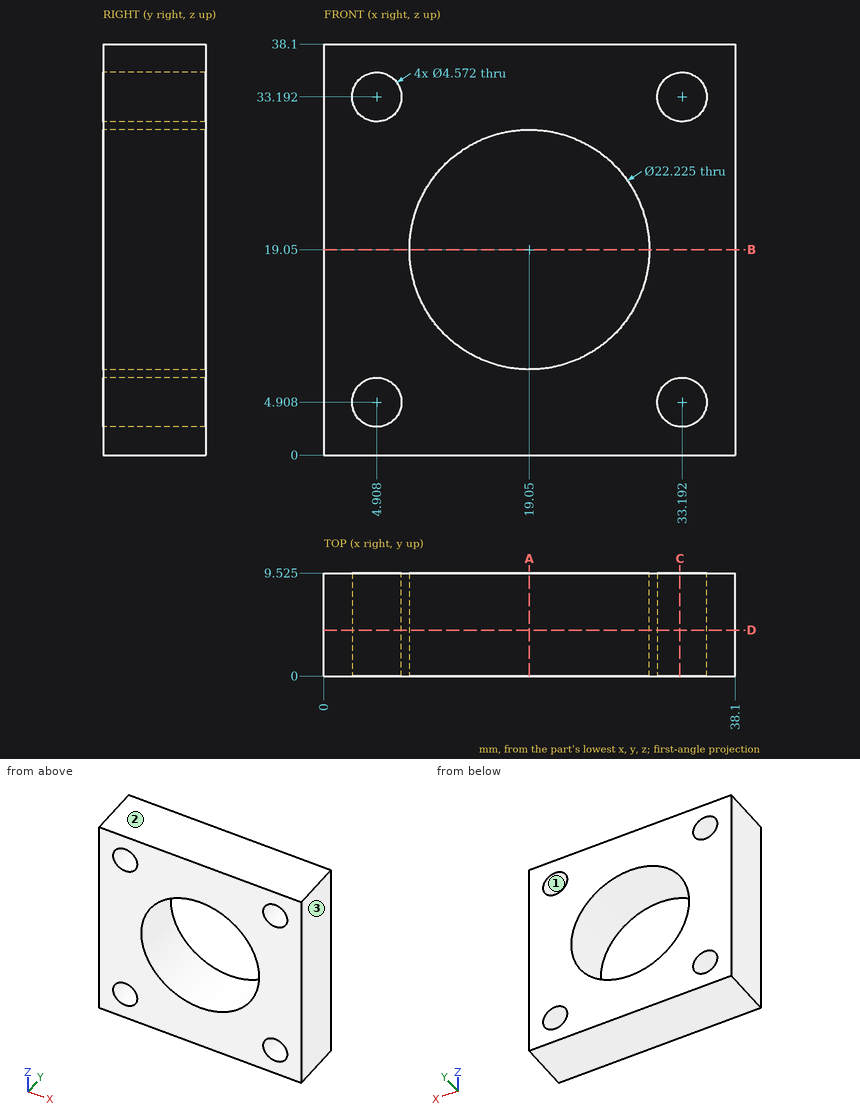
The drawing under review shows one solid part. Ordinate dimensions are in mm from its lowest x, y, z. Coordinates: 2 decimals unless noted, no trailing zeros. Order: outer loops, then holes, each group sorted by start corner. A loop starts at its lowest first (then second) coordinate and runs counter-clockwise, first axis right, second up. Notation, with made-up numbers: (-27.75, 10.5) -> (-6.75, 10.5) arc R22 ccw to (-6.75, 19.5) -> close; hole circle Ø1 at (9, 59). An arc over 180 degrees is marked (long way). Use CSV: the item, a comma, the result in double quotes. Start each with the question number.
Item 1: We need section C-C, the plane x = 33. Give the boundary of the cut face in (y, z) (1 decimal), then the cut area to 3 significant figures.
Item 2: Wall thickness on probe 1 along X at (y, z) = (1, 4); probe 2 along Z at (x, y) = (7, 6); probe 3 along Z at (x, y) = (19.05, 3): over which ranges is each line inside the solid? List them lowest first.
Item 3: We need section D-D, the plane y = 4.25. Give the number of separate pieces and of enclosed holes in the cut face, then the cut area to 3 significant figures.
Item 4: Insertion check: pin 1 (5.5 mm diameter, centred on x = 4.91, z = 33.19, fed in from -Y). The pin has a flat end and moves straight along its axis. Give the tip position at first contact, or say it passes through.
Item 5: Draft analysis for pull direction X (two halves, no side actions). For the marked faces 1, 2 and 3, state which applies: pulls with the +X half, pulls with the -X half, needs draft (parallel to the pull), parting line crosses it, or undercut.
Item 6: We need section A-A, the plane x = 19.05. Give the boundary of the cut face in (y, z) (1 decimal), then the cut area to 3 significant figures.
Item 7: We need section B-B, the plane z = 19.05. Give the boundary of the cut face in (x, y) (1 decimal), then the cut area to 3 significant figures.
Derived:
1,outline,"(0, 0) -> (9.5, 0) -> (9.5, 2.6) -> (0, 2.6) -> close; (0, 7.2) -> (9.5, 7.2) -> (9.5, 30.9) -> (0, 30.9) -> close; (0, 35.5) -> (9.5, 35.5) -> (9.5, 38.1) -> (0, 38.1) -> close"
1,area,"276 mm^2"
2,probe 1,"x = 0 to 2.81, 7.01 to 31.09, 35.29 to 38.1"
2,probe 2,"z = 0 to 3.99, 5.83 to 32.27, 34.11 to 38.1"
2,probe 3,"z = 0 to 7.94, 30.16 to 38.1"
3,separate pieces,"1"
3,enclosed holes,"5"
3,area,"998 mm^2"
4,pin 1,"stops at y = 0"
5,face 1,"undercut"
5,face 2,"needs draft"
5,face 3,"pulls with the +X half"
6,outline,"(0, 0) -> (9.5, 0) -> (9.5, 7.9) -> (0, 7.9) -> close; (0, 30.2) -> (9.5, 30.2) -> (9.5, 38.1) -> (0, 38.1) -> close"
6,area,"151 mm^2"
7,outline,"(0, 0) -> (7.9, 0) -> (7.9, 9.5) -> (0, 9.5) -> close; (30.2, 0) -> (38.1, 0) -> (38.1, 9.5) -> (30.2, 9.5) -> close"
7,area,"151 mm^2"
